```python
from build123d import *

# Parameters (mm, degrees)
ESQUISSE1_R             = 105
ESQUISSE1_R_2           = 4
ESQUISSE1_W             = 30
ESQUISSE1_H             = 70
BOSS_EXTRU_1_DEPTH      = 5
ESQUISSE2_R             = 1.5
ENL_V_MAT_EXTRU_1_DEPTH = 149.576579581
CONG_1_R                = 1
ENL_V_START             = -3
ENL_V_MAT_EXTRU_2_DEPTH = 3
ESQUISSE4_R             = 10
ENL_V_MAT_EXTRU_3_DEPTH = 149.576579581


with BuildPart() as part:
    # Esquisse1 → Boss.-Extru.1 (new body)
    with BuildSketch(Plane.XY):
        Circle(ESQUISSE1_R)
        with Locations((-80, 50)):
            Circle(ESQUISSE1_R_2, mode=Mode.SUBTRACT)
        with Locations(Location((80, 50, 0), (0, 0, 180))):
            Circle(ESQUISSE1_R_2, mode=Mode.SUBTRACT)
        with Locations((80, -50)):
            Circle(ESQUISSE1_R_2, mode=Mode.SUBTRACT)
        with Locations(Location((-80, -50, 0), (0, 0, 180))):
            Circle(ESQUISSE1_R_2, mode=Mode.SUBTRACT)
        with Locations((-80, 0)):
            Rectangle(ESQUISSE1_W, ESQUISSE1_H, mode=Mode.SUBTRACT)
        with Locations((80, 0)):
            Rectangle(ESQUISSE1_W, ESQUISSE1_H, mode=Mode.SUBTRACT)
    extrude(amount=BOSS_EXTRU_1_DEPTH)

    # Esquisse2 → Enlèv. mat.-Extru.1 (cut, through all)
    with BuildSketch(Plane.XY.offset(5)):
        with Locations((-53.5, -8.042853971)):
            Circle(ESQUISSE2_R)
        with Locations((-40, -8.042853971)):
            Circle(ESQUISSE2_R)
        with Locations((-53.5, 8.042853971)):
            Circle(ESQUISSE2_R)
        with Locations((-40, 8.042853971)):
            Circle(ESQUISSE2_R)
        with Locations(Location((40, 8.042853971, 0), (0, 0, 180))):
            Circle(ESQUISSE2_R)
        with Locations(Location((53.5, 8.042853971, 0), (0, 0, 180))):
            Circle(ESQUISSE2_R)
        with Locations(Location((40, -8.042853971, 0), (0, 0, 180))):
            Circle(ESQUISSE2_R)
        with Locations(Location((53.5, -8.042853971, 0), (0, 0, 180))):
            Circle(ESQUISSE2_R)
    extrude(amount=-ENL_V_MAT_EXTRU_1_DEPTH, mode=Mode.SUBTRACT)

    # Congé1
    cong_1_edges = [part.edges().sort_by_distance(p)[0] for p in [
        (95, -35, 2.5),
        (95, 35, 2.5),
        (65, 35, 2.5),
        (65, -35, 2.5),
        (-65, -35, 2.5),
        (-65, 35, 2.5),
        (-95, 35, 2.5),
        (-95, -35, 2.5),
    ]]
    fillet(cong_1_edges, radius=CONG_1_R)

    # Esquisse3 → Enlèv. mat.-Extru.2 (cut)
    with BuildSketch(Plane.XY.offset(5).offset(ENL_V_START)):
        with BuildLine():
            ThreePointArc((24.687033564, 102.056603774), (0, 105), (-24.687033564, 102.056603774))
            Line((-24.687033564, 102.056603774), (-24.687033564, 84.056603774))
            ThreePointArc((-24.687033564, 84.056603774), (0, 63), (24.687033564, 84.056603774))
            Line((24.687033564, 84.056603774), (24.687033564, 102.056603774))
        make_face()
        with BuildLine():
            ThreePointArc((24.687033564, -84.056603774), (0, -63), (-24.687033564, -84.056603774))
            Line((-24.687033564, -84.056603774), (-24.687033564, -102.056603774))
            ThreePointArc((-24.687033564, -102.056603774), (0, -105), (24.687033564, -102.056603774))
            Line((24.687033564, -102.056603774), (24.687033564, -84.056603774))
        make_face()
    extrude(amount=ENL_V_MAT_EXTRU_2_DEPTH, mode=Mode.SUBTRACT)

    # Esquisse4 → Enlèv. mat.-Extru.3 (cut, through all)
    with BuildSketch(Plane.XY.offset(5)):
        with Locations((0, 88)):
            Circle(ESQUISSE4_R)
        with Locations((0, -88)):
            Circle(ESQUISSE4_R)
    extrude(amount=-ENL_V_MAT_EXTRU_3_DEPTH, mode=Mode.SUBTRACT)


solid = part.part
```
Geometry check sheet. Reference: the model listing, model coordinates, mm. A direction names the side the tool comes from. Give positions to 0.01 mm unless a question says otherwise; leave off trailing zeros. Order: outer loops, then holes, each group sorted by start corner. A loop starts at its lowest first (then second) coordinate and runs counter-clockwise, first axis right, second up.
1. Thickness scan on L1, parallel to X at y = -1, z = 1.5; L2, parallel to X at y = -34.5, z = 4.05; L3, parallel to Y at x = -40, z = 3.35. Record the ranges inside material, lowest first.
2. Section check B-B, the plane x = 91. Enter the section's corners in (y, z).
3. Gauge pin test, flat ends, axial feed: pin 1 Ø1.8 at (x, y) = (40, 8.04) entering from -Z; pin 2 Ø1.5 at (y, z) = (7.5, 2.5) entering from -X; pin 3 Ø1.5 at (y, z) = (96.5, 4) entering from -X; pin 4 Ø1 at (x, z) = (-20.5, 0.5) entering from +Y. Record the tip position at first contact, or that the pin passes through.
4. Section check C-C, the plane y = -50. Enter the section's corners in (x, z), and give its area (3 significant figures).
5. Release check for a two-part mould opening along X. For faces 4 (the face through (-1, 1, 5)), 5 (the face through (100.15, 31.54, 2.46)), 6 (the face through (0, 63, 3)) record: pulls with the +X half, pulls with the -X half, needs draft (parallel to the pull), parting line crosses it, or undercut.
6. Access from +Z, -Z, +X, -X, +Y, -Y to the whole of each face (thin tool, end or side, straight path). Record for faces 1 (the face through (0, -63, 3)), 2 (the face through (-5.8, 79.6, 2)), 3 (the face through (80, 35, 2)).
7. Section check D-D, the plane x = -15.5. Enter the section's corners in (y, z), and give its area (3 significant figures).
8. Section check A-A, the plane y = 88. Enter the section's corners in (x, z), and give its area (3 significant figures).
Values follow:
1. L1: x = -105 to -95, -65 to 65, 95 to 105
1. L2: x = -99.17 to -94.87, -65.13 to 65.13, 94.87 to 99.17
1. L3: y = -97.08 to -9.54, -6.54 to 6.54, 9.54 to 97.08
2. outline: (-52.38, 0) - (-35, 0) - (-35, 5) - (-52.38, 5) - close; (35, 0) - (52.38, 0) - (52.38, 5) - (35, 5) - close
3. pin 1: passes through
3. pin 2: stops at x = -104.78
3. pin 3: stops at x = -43.09
3. pin 4: stops at y = 103.08
4. outline: (-92.33, 0) - (-84, 0) - (-84, 5) - (-92.33, 5) - close; (-76, 0) - (76, 0) - (76, 5) - (-76, 5) - close; (84, 0) - (92.33, 0) - (92.33, 5) - (84, 5) - close
4. area: 843 mm2
5. face 4: needs draft
5. face 5: parting line crosses it
5. face 6: undercut
6. face 1: +Z, -Y
6. face 2: +Z, +Y
6. face 3: +Z, -Z
7. outline: (-103.85, 0) - (103.85, 0) - (103.85, 2) - (68.38, 2) - (68.38, 5) - (-68.38, 5) - (-68.38, 2) - (-103.85, 2) - close
7. area: 826 mm2
8. outline: (-57.28, 0) - (-10, 0) - (-10, 2) - (-24.69, 2) - (-24.69, 5) - (-57.28, 5) - close; (10, 0) - (57.28, 0) - (57.28, 5) - (24.69, 5) - (24.69, 2) - (10, 2) - close
8. area: 385 mm2
